Drawing for the job (mm, zero at the part's lowest x, y, z). Give positions to 0.01 mm unless a question says otherwise; leave off trailing zeros. Loops run counter-clockwise (first coordinate to the right, second up) from the corner with the lowest first, then second, coordinate; pieces in that order, holes last. Notation, with made-up numbers: (81.5, 55.5) - (110.5, 55.5) arc R22 cw to (110.5, 86.5) - close; hole circle Ø11 at (24.25, 2.5). An arc over 180 degrees is marked (long way). Return JSON: item names as keys, results as strings. Group by question number.
1) Slice it at B-B (x = 21). List the corners of the cut face in (y, z).
2) Slice it at A-A (y = 7). List the corners of the cut face in (x, z), and give its area (3 significant figures).
3) Drill centre lines: probe 1 along Z at (x, y) = (25.5, 18.5); probe 2 along X at (y, z) = (7.25, 10.75). Where is each one in solid material? Low to high. Write a range as from..to.
4) Slice it at C-C (y = 17.5). List the corners of the cut face in (x, z), and give its area (3 significant figures).
5) Drop flat-ended pins along their axis: pin 1 (6 mm diameter, centred on x = 22.5, y = 17.5, fed in from +Z); pin 2 (8 mm diameter, centred on x = 13, y = 4, fed in from +Z). Give the stop position or say it passes through.
6) Mould opens along Z. For the marked faces 1, 2 and 3 say: released by +Z, released by -Z, zero draft, split by the parting line, or undercut.
7) Slice it at D-D (x = 2.25). List the corners of the cut face in (y, z), and give its area (3 significant figures).
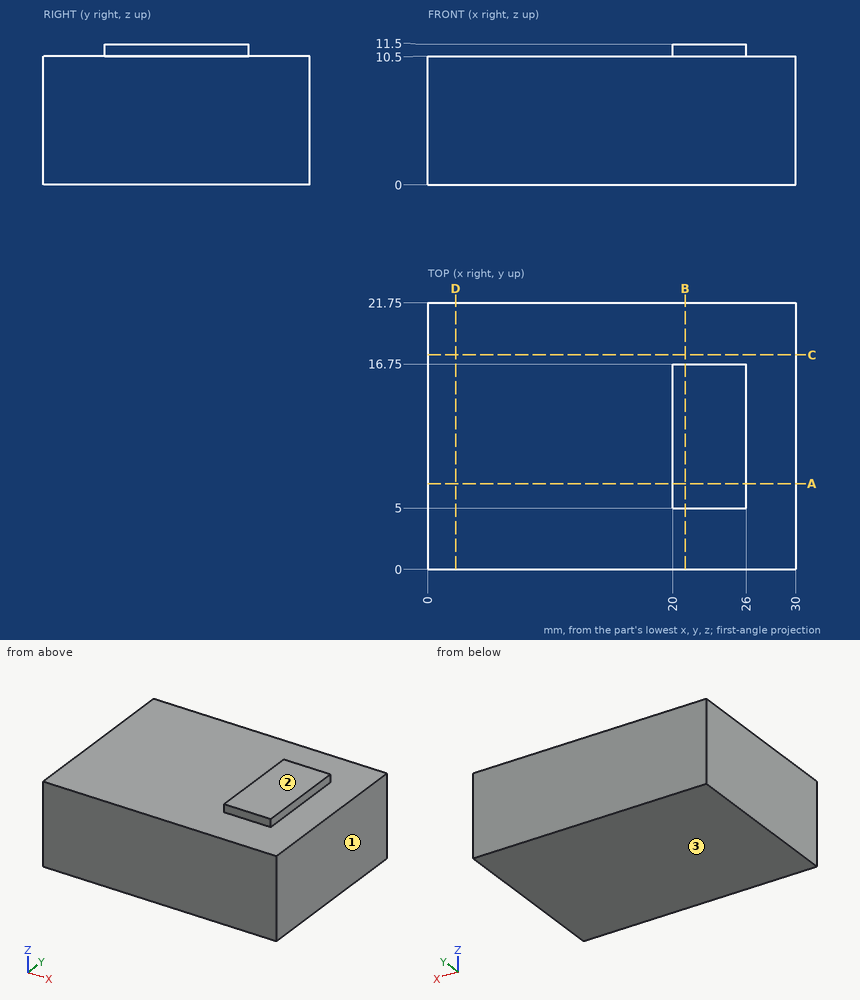
Results:
{
 "1": {"outline": "(0, 0) - (21.75, 0) - (21.75, 10.5) - (16.75, 10.5) - (16.75, 11.5) - (5, 11.5) - (5, 10.5) - (0, 10.5) - close"},
 "2": {"outline": "(0, 0) - (30, 0) - (30, 10.5) - (26, 10.5) - (26, 11.5) - (20, 11.5) - (20, 10.5) - (0, 10.5) - close", "area": "321 mm2"},
 "3": {"probe 1": "0..10.5", "probe 2": "20..26"},
 "4": {"outline": "(0, 0) - (30, 0) - (30, 10.5) - (0, 10.5) - close", "area": "315 mm2"},
 "5": {"pin 1": "z = 11.5", "pin 2": "z = 10.5"},
 "6": {"face 1": "zero draft", "face 2": "released by +Z", "face 3": "released by -Z"},
 "7": {"outline": "(0, 0) - (21.75, 0) - (21.75, 10.5) - (0, 10.5) - close", "area": "228 mm2"}
}
